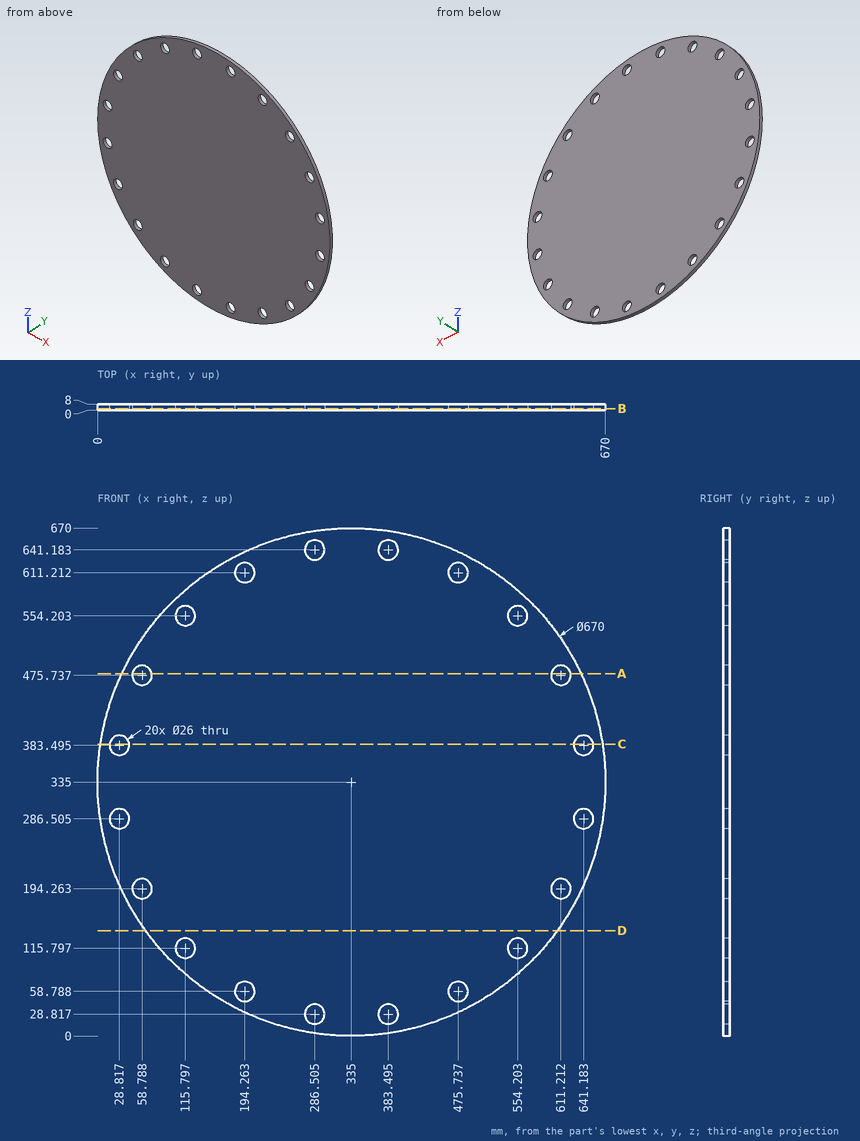
The figure shows three views and two pictorial views of one solid part (mm, origin at its lowest corner). Answer the questions. Round coordinates to 2 decimals unless told otherwise and drop trailing zeros. Write each loop counter-clockwise with the first axis right and the second up, starting at its lowest first coordinate (ties: lowest second). Pieces come first, ordered by that corner, then holes. Notation, with made-up numbers: (8, -22) - (23, -22) arc R32 ccw to (23, 13) - close; hole circle Ø7 at (-16.5, 6.25). An arc over 180 degrees is marked (long way). Use one line per item in the form item = value. Start each with the question number.
Item 1: Flat-ended cylindrical pins translate along their axes: pin 1 Ø4 at (x, y) = (108.5, 3.5) entering from -Z (1 decimal); pin 2 Ø3 at (x, y) = (575, 5.5) entering from -Z; pin 3 Ø23.5 at (x, z) = (58.79, 194.26) entering from +Y; pin 4 Ø1.5 at (x, y) = (490.5, 5) entering from +Z (1 decimal). Find the tip coordinate at first contact, or state that the pin passes through.
Item 2: A cutting plane is placed at A-A (z = 478). Write down the section's boundary in (x, y) (1 decimal), plus the area to 3 significant figures.
Item 3: A cutting plane is placed at B-B (y = 1.75). Give the number of separate pieces and of enclosed holes in the cut face, plus the area to 3 significant figures.
Item 4: A cutting plane is placed at D-D (z = 139). Write down the section's boundary in (x, y), plus the area to 3 significant figures.
Item 5: A cutting plane is placed at C-C (z = 385). Write down the section's boundary in (x, y), plus the area to 3 significant figures.
Item 6: Find the intervals of material crossed by line 1 (X direction, y = 3, z = 280) (1 decimal); line 2 (Z direction, x = 639.5, y = 0.5) (1 decimal); line 3 (X direction, y = 5.5, z = 558) (1 decimal), in increasing order. Write a range as [from, to].
The answers:
q1.pin_1 = 86.4
q1.pin_2 = 99.75
q1.pin_3 = through
q1.pin_4 = 632.1
q2.outline = (32.1, 0) - (46, 0) - (46, 8) - (32.1, 8) - close; (71.6, 0) - (598.4, 0) - (598.4, 8) - (71.6, 8) - close; (624, 0) - (637.9, 0) - (637.9, 8) - (624, 8) - close
q2.area = 4,440 mm^2
q3.separate_pieces = 1
q3.enclosed_holes = 20
q3.area = 342,000 mm^2
q4.outline = (63.32, 0) - (606.68, 0) - (606.68, 8) - (63.32, 8) - close
q4.area = 4,350 mm^2
q5.outline = (3.75, 0) - (15.9, 0) - (15.9, 8) - (3.75, 8) - close; (41.73, 0) - (628.27, 0) - (628.27, 8) - (41.73, 8) - close; (654.1, 0) - (666.25, 0) - (666.25, 8) - (654.1, 8) - close
q5.area = 4,890 mm^2
q6.line_1 = [4.5, 17.6], [40.1, 629.9], [652.4, 665.5]
q6.line_2 = [195.3, 273.6], [299.4, 370.6], [396.4, 474.7]
q6.line_3 = [85, 103.4], [128.2, 541.8], [566.6, 585]
